from build123d import *

# Parameters (mm, degrees)
SKETCH_1_W          = 36
SKETCH_1_H          = 32
SKETCH_1_R          = 1.5
EXTRUDE_1_DEPTH     = 4
EXTRUDE_2_DEPTH     = 32
SKETCH_8_R          = 1.5
CUT_EXTRUDE_1_DEPTH = 5


with BuildPart() as part:
    # Эскиз1 → Бобышка-Вытянуть1 (new body)
    with BuildSketch(Plane.XY):
        with Locations((18, 16)):
            Rectangle(SKETCH_1_W, SKETCH_1_H)
        with Locations((8, 26)):
            Circle(SKETCH_1_R, mode=Mode.SUBTRACT)
        with Locations((28, 26)):
            Circle(SKETCH_1_R, mode=Mode.SUBTRACT)
        with Locations((8, 6)):
            Circle(SKETCH_1_R, mode=Mode.SUBTRACT)
        with Locations((28, 6)):
            Circle(SKETCH_1_R, mode=Mode.SUBTRACT)
    extrude(amount=EXTRUDE_1_DEPTH)

    # Эскиз7 → Бобышка-Вытянуть2 (add)
    with BuildSketch(Plane(origin=(0, 32, 0), x_dir=(1, 0, 0), z_dir=(0, 1, 0))):
        Polygon((0, 0), (-1.2, 0), (-1.2, 15), (-5.2, 15), (-5.2, -19), (-1.2, -19), (-1.2, -4), (0, -4), align=None)
    extrude(amount=-EXTRUDE_2_DEPTH)

    # Эскиз8 → Вырез-Вытянуть1 (cut, through all)
    with BuildSketch(Plane(origin=(-1.2, 0, 0), x_dir=(0, 0, -1), z_dir=(1, 0, 0))):
        with Locations((8, 24)):
            Circle(SKETCH_8_R)
        with Locations((8, 8)):
            Circle(SKETCH_8_R)
        with Locations((-12, 8)):
            Circle(SKETCH_8_R)
        with Locations((-12, 24)):
            Circle(SKETCH_8_R)
    extrude(amount=-CUT_EXTRUDE_1_DEPTH, mode=Mode.SUBTRACT)


solid = part.part
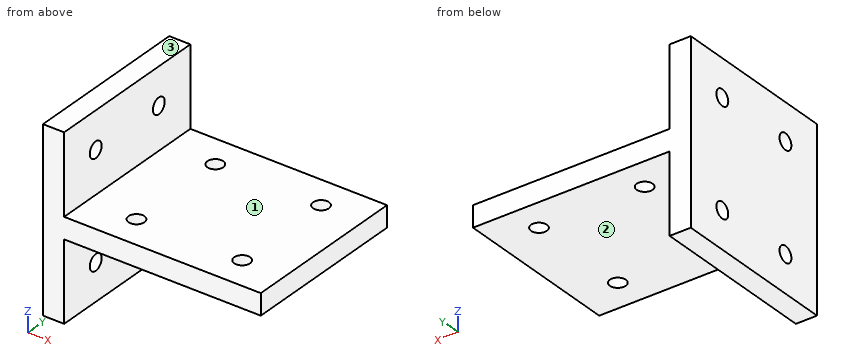
Check sheet for the modelled part. Datum: model origin and axes. Units: mm. Face numbers are marked on the shaded views. A direction names the side the tool comes from. Give positions to 0.01 mm unless a question says otherwise; leave off trailing zeros. Write each loop counter-clockwise with the first axis right and the second up, starting at its lowest first coordinate (ties: lowest second). Pieces come first, ordered by that corner, then holes. Notation, with made-up numbers: (-38.75, 47) -> (11.25, 47) arc R22 cw to (11.25, 53) -> close; hole circle Ø6 at (69.25, 44.5). An arc over 180 degrees is marked (long way). One line per item, written item: value. Start each with the question number.
Item 1: Section check C-C on y = 8. Record the cut outline in (x, z).
Item 2: Section check B-B on x = 28. Record the cut outline in (y, z), then the cut area to 3 significant figures.
Item 3: Tool access check on the marked faces 1, 2 and 3. Record the directions out of +Z, -Z, +X, -X, +Y, -Y that give a thin tool (end or side, any length) a straight path to the whole face; none if there is none.
Item 4: Section check A-A on z = 0.5. Record the cut outline in (x, y).
Item 5: Material ranges on probe 1 along Y at (x, z) = (28, 2.85); probe 2 along Y at (x, z) = (-3, -8); probe 3 along X at (y, z) = (14.5, -3), recorded low to high. Write a range as from..to.
Item 6: Section check D-D on z = 12. Record the cut outline in (x, y), then the cut area to 3 significant figures.
Item 7: Gauge pin test, flat ends, axial feed: pin 1 (12 mm diameter, centred on x = 27.5, y = 6.5, fed in from -Z); pin 2 (9.5 mm diameter, centred on x = 26.5, y = 11.5, fed in from +Z); pin 3 (4.5 mm diameter, centred on y = 23.5, z = 11, fed in from +X). Record the tip position at first contact, or that the pin passes through.
Results list:
1. outline: (-5.2, -15) -> (-1.2, -15) -> (-1.2, -9.5) -> (-5.2, -9.5) -> close; (-5.2, -6.5) -> (-1.2, -6.5) -> (-1.2, 0) -> (36, 0) -> (36, 4) -> (-1.2, 4) -> (-1.2, 10.5) -> (-5.2, 10.5) -> close; (-5.2, 13.5) -> (-1.2, 13.5) -> (-1.2, 19) -> (-5.2, 19) -> close
2. outline: (0, 0) -> (4.5, 0) -> (4.5, 4) -> (0, 4) -> close; (7.5, 0) -> (24.5, 0) -> (24.5, 4) -> (7.5, 4) -> close; (27.5, 0) -> (32, 0) -> (32, 4) -> (27.5, 4) -> close
2. area: 104 mm²
3. face 1: +Z, +X, +Y, -Y
3. face 2: -Z, +X, +Y, -Y
3. face 3: +Z, +X, -X, +Y, -Y
4. outline: (-5.2, 0) -> (36, 0) -> (36, 32) -> (-5.2, 32) -> close; hole circle Ø3 at (8, 6); hole circle Ø3 at (8, 26); hole circle Ø3 at (28, 6); hole circle Ø3 at (28, 26)
5. probe 1: 0..4.5, 7.5..24.5, 27.5..32
5. probe 2: 0..6.5, 9.5..22.5, 25.5..32
5. probe 3: -5.2..-1.2
6. outline: (-5.2, 0) -> (-1.2, 0) -> (-1.2, 6.5) -> (-5.2, 6.5) -> close; (-5.2, 9.5) -> (-1.2, 9.5) -> (-1.2, 22.5) -> (-5.2, 22.5) -> close; (-5.2, 25.5) -> (-1.2, 25.5) -> (-1.2, 32) -> (-5.2, 32) -> close
6. area: 104 mm²
7. pin 1: z = 0
7. pin 2: z = 4
7. pin 3: x = -1.2
